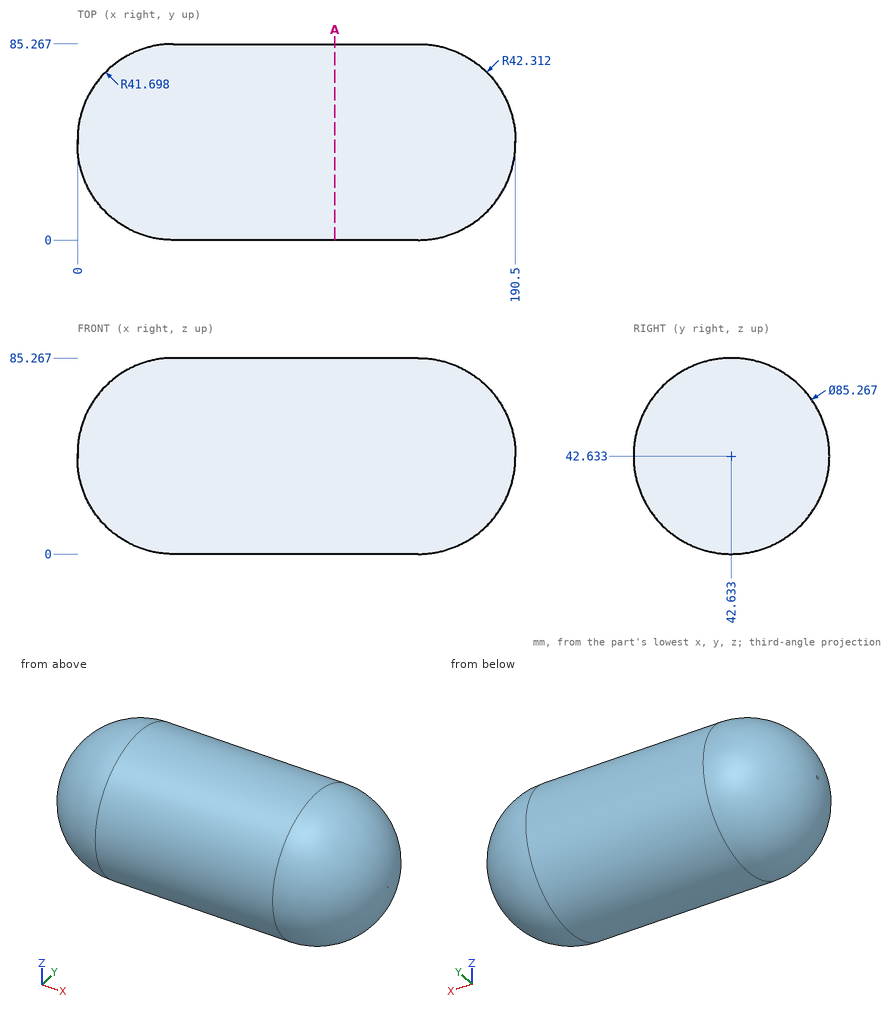
Study the drawing (mm; zero at the part's minimum x, y, z) and answer. Round coordinates to 2 decimals unless told otherwise and drop trailing zeros. Loops run counter-clockwise (first coordinate to the right, second up) from the corner with the lowest first, then second, coordinate; pieces in that order, holes last. Notation, with made-up numbers: (47, 23.5) -> (70, 23.5) arc R11 cw to (70, 35.5) -> close; hole circle Ø6 at (-31, 24). An arc over 180 degrees is marked (long way). Write each question's results on one line, items separated by ' | '. Start each with the question number.
1. Given pin 1 Ø2 at (y, z) = (11, 67.5) entering from -X (1 decimal); pin 2 Ø10 at (x, y) = (97.5, 43) entering from -Z; pin 3 Ø6 at (x, y) = (158.5, 21.5) entering from +Z, each flat-ended and moving along its own axis, determine where each tip first touches the part or whether it passes through.
2. Section A-A (x = 112) is taken. Determine the outline of the cut face in (y, z).
3. Find the intervals of material crossed by probe 1 along Z at (x, y) = (85, 5) (1 decimal); probe 2 along Y at (x, z) = (82.5, 9) (1 decimal); probe 3 along Z at (x, y) = (147, 16.5), in increasing order. Write a range as from..to.
Evaluation:
1) pin 1: stops at x = 25.2 | pin 2: stops at z = 0 | pin 3: stops at z = 80
2) outline: circle Ø85.27 at (42.63, 42.63)
3) probe 1: z = 22.6..62.7 | probe 2: y = 16.4..68.8 | probe 3: z = 8.95..76.32
